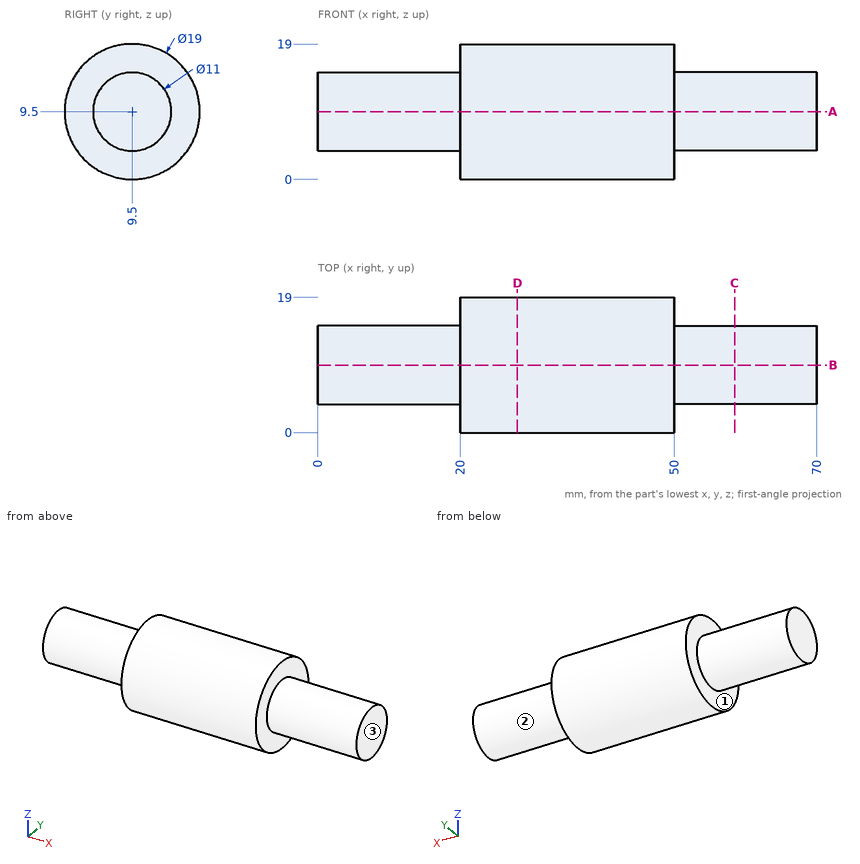
Study the drawing (mm; zero at the part's minimum x, y, z) and answer. A direction names the side the tool comes from. Coordinates: 2 decimals unless noted, no trailing zeros. Write each loop counter-clockwise with the first axis right and the second up, starting at its lowest first coordinate (ties: lowest second). Pieces come first, ordered by that corner, then holes. Notation, with made-up numbers: (83.5, 16) - (125.5, 16) arc R22 ccw to (125.5, 43) - close; hole circle Ø4 at (-39.75, 15.25). An arc over 180 degrees is marked (long way). Answer as a JSON object with one key per item and string values. Group by question number.
1. Which of the six approach directions +Z, -Z, +X, -X, +Y, -Y give full straight-line access (tool end or side, diameter ignored) to the marked faces 1, 2 and 3?
2. A cutting plane is placed at A-A (z = 9.5). Determine the outline of the cut face in (x, y), plus the area to 3 significant figures.
3. Consider L1, parallel to X at y = 1.5, z = 8.75; L2, parallel to Z at x = 28, y = 1.75; L3, parallel to Y at x = 31, z = 10. Determine where each line is inside the solid, lowest interval first. Write a range as [from, to].
4. A cutting plane is placed at C-C (x = 58.5). Determine the outline of the cut face in (y, z).
5. Each of these flat-tipped pins is pushed along its axis until it touches: P1, Ø2, axis at x = 34, z = 15, coming from the -Y side; P2, Ø2, axis at x = 35.5, y = 7, coming from the -Z side; P3, Ø5, axis at x = 50, y = 2.5, coming from the +Z side. Where does it stop, or does it pass through?
6. A cutting plane is placed at D-D (x = 28). Determine the outline of the cut face in (y, z), plus the area to 3 significant figures.
Worked out:
{
 "1": {"face 1": "-X", "face 2": "+X", "face 3": "+Z, -Z, +X, +Y, -Y"},
 "2": {"outline": "(0, 4) - (20, 4) - (20, 0) - (50, 0) - (50, 4) - (70, 4) - (70, 15) - (50, 15) - (50, 19) - (20, 19) - (20, 15) - (0, 15) - close", "area": "1,010 mm²"},
 "3": {"L1": "x = [20, 50]", "L2": "z = [4.01, 14.99]", "L3": "y = [0.01, 18.99]"},
 "4": {"outline": "circle Ø11 at (9.5, 9.5)"},
 "5": {"P1": "stops at y = 1.13", "P2": "stops at z = 0.12", "P3": "stops at z = 17.87"},
 "6": {"outline": "circle Ø19 at (9.5, 9.5)", "area": "284 mm²"}
}
